CAD build for the part. Positions are in the model's coordinates, mm. Face numbers are marked on the shaded views. A direction names the side the tool comes from. Round coordinates to 2 decimals unless told otherwise and drop trailing zeros. Order: outer loops, then holes, each group sorted by start corner. A loop starts at its lowest first (then second) coordinate and runs counter-clockwise, first axis right, second up. Notation, with made-up numbers: M 88.25,33.25 L 128.25,33.25 A29 cw 128.25,57.25 Z; hole C 7,76 d4. An arc over 180 degrees is marked long. Put each result on its own line as item: value.
```python
from build123d import *

# Parameters (mm, degrees)
SKETCH_W         = 70
SKETCH_H         = 70
PAD_DEPTH        = 45
SKETCH001_R      = 35
PAD001_DEPTH     = 100
POCKET_DEPTH     = 70
REVOLUTION_ANGLE = -180
SKETCH004_R      = 20.5
PAD002_DEPTH     = 14
SKETCH005_R      = 10
PAD003_DEPTH     = 14.5
PAD004_DEPTH     = 14
SKETCH007_R      = 3
POCKET001_DEPTH  = 10


with BuildPart() as part:
    # Sketch → Pad (new body)
    with BuildSketch(Plane.XY):
        with Locations((0, 35)):
            Rectangle(SKETCH_W, SKETCH_H)
    extrude(amount=PAD_DEPTH)

    # Sketch001 → Pad001 (new body)
    with BuildSketch(Plane.XY.offset(45)):
        with Locations((0, 35)):
            Circle(SKETCH001_R)
    extrude(amount=PAD001_DEPTH)

    # Sketch002 → Pocket (cut)
    with BuildSketch(Plane(origin=(0, 0, 0), x_dir=(1, 0, 0), z_dir=(0, 0, -1))):
        Polygon((35, 0), (35, -3), (32, 0), align=None)
        Polygon((35, -70), (35, -67), (32, -70), align=None)
        Polygon((-35, -70), (-32, -70), (-35, -67), align=None)
        Polygon((-35, 0), (-32, 0), (-35, -3), align=None)
    extrude(amount=-POCKET_DEPTH, mode=Mode.SUBTRACT)

    # Sketch003 → Revolution (revolve)
    with BuildSketch(Plane.XY.offset(145)):
        with BuildLine():
            ThreePointArc((0, 0), (35, 35), (0, 70))
            Line((0, 70), (0, 0))
        make_face()
    revolve(axis=Axis((0, 0, 145), (0, 1, 0)), revolution_arc=REVOLUTION_ANGLE)

    # Sketch004 → Pad002 (new body)
    with BuildSketch(Plane(origin=(0, 0, 0), x_dir=(1, 0, 0), z_dir=(0, 0, -1))):
        with Locations((0, -35)):
            Circle(SKETCH004_R)
    extrude(amount=PAD002_DEPTH)

    # Sketch005 → Pad003 (new body)
    with BuildSketch(Plane(origin=(0, 0, -14), x_dir=(1, 0, 0), z_dir=(0, 0, -1))):
        with Locations((0, -35)):
            Circle(SKETCH005_R)
    extrude(amount=PAD003_DEPTH)

    # Sketch006 → Pad004 (new body)
    with BuildSketch(Plane(origin=(0, 0, 0), x_dir=(1, 0, 0), z_dir=(0, 0, -1))):
        Polygon((35, -3), (35, -14.5), (-35, -14.5), (-35, -3), (-32, 0), (32, 0), align=None)
    extrude(amount=PAD004_DEPTH)

    # Sketch007 → Pocket001 (cut)
    with BuildSketch(Plane.XZ):
        Circle(SKETCH007_R)
    extrude(amount=-POCKET001_DEPTH, mode=Mode.SUBTRACT)


solid = part.part
```
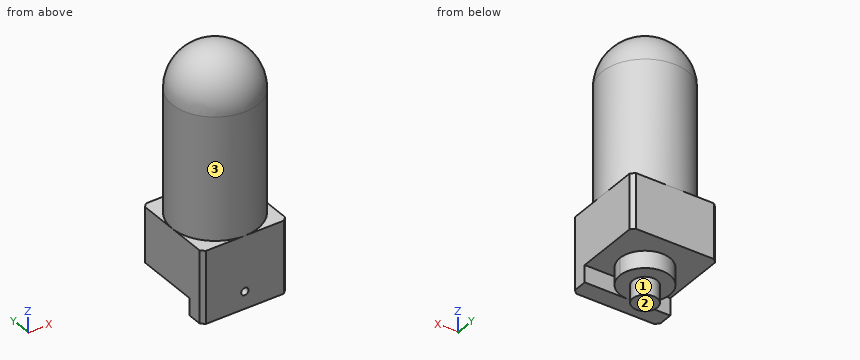
Item 1: Band-saw the part on B-B on z = 64. Give the cut face in (x, y), and give its area (3 significant figures).
Answers below:
outline: C 0,35 d70
area: 3,850 mm²
Item 2: Probe line 1 along Y through (x, z) = (-21, -5); line 2 along Z through (x, y) = (0, 3); line 3 along Z through (x, y) = (0, 4). List the from-to ranges inside material, lowest first. Write a range as [from, to].
Answers below:
line 1: [0, 14.5]
line 2: [-14, -3], [3, 159.18]
line 3: [-14, -3], [3, 161.25]
Item 3: Band-saw the part on A-A on x = 25. Give the cut face in (y, z), and give its area (3 significant figures).
Answers below:
outline: M 0,-14 L 14.5,-14 L 14.5,0 L 70,0 L 70,45 L 59.49,45 L 59.49,145 A24.49 ccw 10.51,145 L 10.51,45 L 0,45 Z
area: 9,190 mm²
Item 4: Band-saw the part on C-C on y = 37. Give the cut face in (x, z), and give its area (3 significant figures).
Answers below:
outline: M -35,0 L -20.4,0 L -20.4,-14 L -9.8,-14 L -9.8,-28.5 L 9.8,-28.5 L 9.8,-14 L 20.4,-14 L 20.4,0 L 35,0 L 35,45 L 34.94,45 L 34.94,145 A34.94 ccw -34.94,145 L -34.94,45 L -35,45 Z
area: 12,900 mm²
Item 5: Tool access for the marked faces 1, 2 and 3: list every direction of +Z, -Z, +X, -X, +Y, -Y with a clear straight run to the whole face (end or side of a thin tool).
Answers below:
face 1: -Z
face 2: -Z, +X, -X, +Y, -Y
face 3: +Z
Item 6: Band-saw the part on D-D on x = -15. Give the cut face in (y, z), and give its area (3 significant figures).
Answers below:
outline: M 0,-14 L 14.5,-14 L 14.5,0 L 21.03,0 L 21.03,-14 L 48.97,-14 L 48.97,0 L 70,0 L 70,45 L 66.62,45 L 66.62,145 A31.62 ccw 3.38,145 L 3.38,45 L 0,45 Z
area: 11,600 mm²
Item 7: Pin check, flat tips, straight feed: P1, Ø11, axis at x = -14.5, z = -6.5, coming from the +Y side; P2, Ø2, axis at y = 61.5, z = 115.5, coming from the -X side; P3, Ø12, axis at x = 27, y = 38, coming from the +Z side. Stop position of each tip, or through.
Answers below:
P1: y = 53.42
P2: x = -23.97
P3: z = 172.87
